Here's the drawing with two shaded views (mm, measured from the low corner). I have some questions. Coordinates: 2 decimals unless noted, no trailing zeros. Write each loop counter-clockwise with the first axis right and the second up, starting at its lowest first coordinate (ties: lowest second). Pieces come first, ordered by that corner, then holes. Notation, with made-up numbers: M -36,-18 L -12,-18 A28 ccw -12,11 Z; hole C -23.75,69.25 d10. An arc over 180 degrees is marked long. Answer as CSV lines item,"result". Start each with the question number.
Item 1: Suppose I cut it at B-B, the plane x = 5.5. Write out the boundary of the cut face in (y, z).
Item 2: We'd pull the mould along Y, two halves only. Please class the marked faces 1, 2, 3 and 4: +Y half, -Y half, draft (parallel to the pull), parting line (faces both ways), or undercut.
Item 3: If I drill on line 1 along X through (y, z) = (8.75, 2.4); line 2 along X through (y, z) = (5.5, 0.35); line 3 along Y through (x, z) = (5.5, 1.1), over which ranges is the centre line in solid material (lowest first)? Write a range as [from, to].
Item 4: Suppose I cut it at C-C, the plane z = 2.2. Write out the boundary of the cut face in (x, y), and give its area (3 significant figures).
Item 5: Suppose I cut it at A-A, the plane y = 9. Write out the boundary of the cut face in (x, z), and give its area (3 significant figures).
Item 6: I'm going to push flat-ended pins straight in: P1, Ø5, axis at x = 36.5, y = 15, coming from the +Z side; P2, Ø6.5, axis at x = 27, y = 9, coming from the -Z side. Where does each tip first touch, or does it pass through?
Item 7: Suppose I cut it at D-D, the plane x = 27. Write out the boundary of the cut face in (y, z).
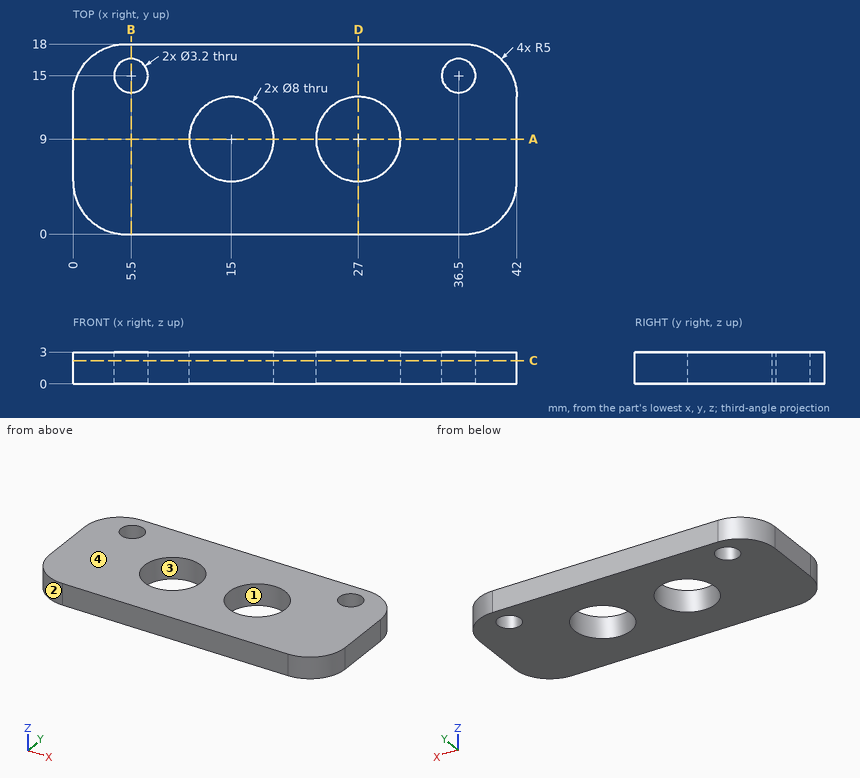
Ans:
1,outline,"M 0,0 L 13.4,0 L 13.4,3 L 0,3 Z; M 16.6,0 L 18,0 L 18,3 L 16.6,3 Z"
2,face 1,"undercut"
2,face 2,"-Y half"
2,face 3,"undercut"
2,face 4,"draft"
3,line 1,"x = [0, 11.01], [18.99, 23.01], [30.99, 42]"
3,line 2,"x = [0, 13.06], [16.94, 25.06], [28.94, 42]"
3,line 3,"y = [0, 13.4], [16.6, 18]"
4,outline,"M 0,5 A5 ccw 5,0 L 37,0 A5 ccw 42,5 L 42,13 A5 ccw 37,18 L 5,18 A5 ccw 0,13 Z; hole C 5.5,15 d3.2; hole C 15,9 d8; hole C 27,9 d8; hole C 36.5,15 d3.2"
4,area,"618 mm^2"
5,outline,"M 0,0 L 11,0 L 11,3 L 0,3 Z; M 19,0 L 23,0 L 23,3 L 19,3 Z; M 31,0 L 42,0 L 42,3 L 31,3 Z"
5,area,"78.0 mm^2"
6,P1,"stops at z = 3"
6,P2,"passes through"
7,outline,"M 0,0 L 5,0 L 5,3 L 0,3 Z; M 13,0 L 18,0 L 18,3 L 13,3 Z"
